CAD build for the part. Positions are in the model's coordinates, mm. A direction names the side the tool comes from. Give positions to 0.01 mm unless a question says otherwise; leave off trailing zeros. Write each loop counter-clockwise with the first axis right and the second up, starting at its lowest first coordinate (ties: lowest second). Pieces come first, ordered by that corner, then holes. Notation, with made-up numbers: (54.25, -36) -> (101.25, -36) arc R10 ccw to (101.25, -25) -> close; hole circle Ø5 at (22.25, 63.5). An arc over 180 degrees is marked (long way). Answer in a Markdown table with one row per item. Add a question column.
```python
from build123d import *

# Parameters (mm, degrees)
SKIZZE1_R                                            = 1.5
AUFSATZ_LINEAR_AUSTRAGEN1_DEPTH                      = 30
AUFSATZ_LINEAR_AUSTRAGEN2_DEPTH                      = 1
VERRUNDUNG1_R                                        = 10
VERRUNDUNG2_R                                        = 12
STIRNSENKUNG_F_R_M3_FLACHKOPFSCHRAUBE_MI_D           = 3.4
STIRNSENKUNG_F_R_M3_FLACHKOPFSCHRAUBE_MI_CBORE_D     = 7
STIRNSENKUNG_F_R_M3_FLACHKOPFSCHRAUBE_MI_CBORE_DEPTH = 2.4


with BuildPart() as part:
    # Skizze1 → Aufsatz-Linear austragen1 (new body)
    with BuildSketch(Plane(origin=(0, 0, 0), x_dir=(1, 0, 0), z_dir=(0, 1, 0))):
        Polygon((-50, 50), (50, 50), (50, -50), (-50, -50), (-50, 35), align=None)
        with Locations(Location((42.5, 42.5, 0), (0, 0, 270))):
            Circle(SKIZZE1_R, mode=Mode.SUBTRACT)
        with Locations(Location((-42.5, 42.5, 0), (0, 0, 270))):
            Circle(SKIZZE1_R, mode=Mode.SUBTRACT)
        with Locations(Location((42.5, -42.5, 0), (0, 0, 270))):
            Circle(SKIZZE1_R, mode=Mode.SUBTRACT)
        with Locations(Location((-42.5, -42.5, 0), (0, 0, 270))):
            Circle(SKIZZE1_R, mode=Mode.SUBTRACT)
        Polygon((-47, -35), (-35, -35), (-35, -47), (35, -47), (35, -35), (47, -35), (47, 35), (35, 35), (35, 47), (-35, 47), (-35, 35), (-47, 35), align=None, mode=Mode.SUBTRACT)
    extrude(amount=-AUFSATZ_LINEAR_AUSTRAGEN1_DEPTH)

    # Skizze1<3> → Aufsatz-Linear austragen2 (add)
    with BuildSketch(Plane(origin=(0, 0, 0), x_dir=(1, 0, 0), z_dir=(0, 1, 0))):
        Polygon((35, 47), (-35, 47), (-35, 35), (-47, 35), (-47, -35), (-35, -35), (-35, -47), (35, -47), (35, -35), (47, -35), (47, 35), (35, 35), align=None)
        Polygon((-7.8359, -3.0607), (-6.9977, -3.0607), (-6.9977, 3.0607), (-7.8359, 3.0607), (-7.8359, 6.9977), (-6.9977, 6.9977), (6.9977, 6.9977), (7.8359, 6.9977), (7.8359, 3.0607), (6.9977, 3.0607), (6.9977, -3.0607), (7.8359, -3.0607), (7.8359, -6.9977), (6.9977, -6.9977), (-6.9977, -6.9977), (-7.8359, -6.9977), align=None, mode=Mode.SUBTRACT)
    extrude(amount=-AUFSATZ_LINEAR_AUSTRAGEN2_DEPTH)

    # Verrundung1
    verrundung1_edges = [part.edges().sort_by_distance(p)[0] for p in [
        (50, -15, -50),
        (50, -15, 50),
        (-50, -15, 50),
        (-50, -15, -50),
    ]]
    fillet(verrundung1_edges, radius=VERRUNDUNG1_R)

    # Verrundung2
    verrundung2_edges = [part.edges().sort_by_distance(p)[0] for p in [
        (35, -15.5, 35),
        (-35, -15.5, 35),
        (35, -15.5, -35),
        (-35, -15.5, -35),
    ]]
    fillet(verrundung2_edges, radius=VERRUNDUNG2_R - 0.0001)  # a hair under: the kernel refuses the full size

    # Stirnsenkung für M3 Flachkopfschraube mit Schlitz1 (through all)
    with Locations(Plane(origin=(0, 0, 0), x_dir=(1, 0, 0), z_dir=(0, 1, 0))):
        with Locations((-42.5, -42.5), (-42.5, 42.5), (42.5, -42.5), (42.5, 42.5)):
            CounterBoreHole(STIRNSENKUNG_F_R_M3_FLACHKOPFSCHRAUBE_MI_D / 2, STIRNSENKUNG_F_R_M3_FLACHKOPFSCHRAUBE_MI_CBORE_D / 2, STIRNSENKUNG_F_R_M3_FLACHKOPFSCHRAUBE_MI_CBORE_DEPTH)

    # Skizze9 → Rotation1 (revolve)
    with BuildSketch(Plane.XY):
        Polygon((45.009357924, 0), (42.120640981, 11.470793218), (36.483893338, 11.470793218), (36.483893338, 0), align=None)
    revolve(axis=Axis((0, -1000, 0), (0, 1, 0)))


solid = part.part
```
Item 1: Mould opens along X. For faces 1 (the face through (46.99, -15.21, -47.15)), 2 (the face through (39.92, -1.183, 40.135)), 3 (the face through (-46.99, -15.21, -47.15)) say: released by +X, released by -X, zero draft, split by the parting line, or undercut.
Item 2: Drop flat-ended pins along their axis: pin 1 Ø2 at (x, y) = (-17.5, 3.5) entering from -Z; pin 2 Ø3 at (y, z) = (2, -8.5) entering from -X; pin 3 Ø3 at (x, z) = (42.5, 42.5) entering from +Y; pin 4 Ø4 at (x, z) = (-42.5, 42.5) entering from -Y. Give the stop position or say it passes through.
Item 3: Which spindle directions (+Z, -Z, +X, -X, +Y, -Y) get a long thin tool onto all of the face, cutting with end or side? Do faces 4 (the face through (47, -15, 0)), 5 (the face through (-36.45, 5.66, -1.6)), 6 (the face through (-41.15, -16.39, -41.47)). Say none if no direction does.
Item 4: Slice it at A-A, the plane y = -7.5. State how many separate pieces and enclosed holes the cut face has, then the cut area to 3 significant figures.
Item 5: Probe L1, parallel to X at y = -15, z = -10; L2, parallel to Z at x = -43, y = -24; L3, parallel to X at y = -0.65, z = -42.5. List the from-to ranges inside material, lowest first. Write a range as from..to.
Item 6: Slice it at B-B, the plane x = 0. List the corners of the cut face in (y, z), then the cut area to 3 significant figures.
Answer key:
| question | item | result |
|---|---|---|
| 1 | face 1 | released by +X |
| 1 | face 2 | undercut |
| 1 | face 3 | released by -X |
| 2 | pin 1 | stops at z = -41.01 |
| 2 | pin 2 | stops at x = -44.16 |
| 2 | pin 3 | passes through |
| 2 | pin 4 | stops at y = -30 |
| 3 | face 4 | -Y |
| 3 | face 5 | +Y |
| 3 | face 6 | +Y, -Y |
| 4 | separate pieces | 1 |
| 4 | enclosed holes | 5 |
| 4 | area | 1,490 mm² |
| 5 | L1 | x = -50..-47, 47..50 |
| 5 | L2 | z = -49.54..-44.12, -40.88..-35.69, 35.69..40.88, 44.12..49.54 |
| 5 | L3 | x = -49.68..-46, -39..39, 46..49.68 |
| 6 | outline | (-30, -50) -> (0, -50) -> (0, -45.01) -> (11.47, -42.12) -> (11.47, -36.48) -> (0, -36.48) -> (0, -7) -> (-1, -7) -> (-1, -47) -> (-30, -47) -> close; (-30, 47) -> (-1, 47) -> (-1, 7) -> (0, 7) -> (0, 36.48) -> (11.47, 36.48) -> (11.47, 42.12) -> (0, 45.01) -> (0, 50) -> (-30, 50) -> close |
| 6 | area | 422 mm² |
